```python
from build123d import *

# Parameters (mm, degrees)
PAD_DEPTH   = 40
SKETCH001_R = 7
HOLE_DEPTH  = 12.001


with BuildPart() as part:
    # Sketch → Pad (new body)
    with BuildSketch(Plane.XZ):
        Polygon((0, 0), (-18, 0), (-18, 7), (-13, 7), (-13, 2.5), (-10.5, 2.5), (-10.5, 9.5), (-20.5, 9.5), (-20.5, 12), (20.5, 12), (20.5, 9.5), (10.5, 9.5), (10.5, 2.5), (13, 2.5), (13, 7), (18, 7), (18, 0), align=None)
    extrude(amount=PAD_DEPTH)

    # Sketch001 (on Face9 of Pad) → Hole (cut, through all)
    with BuildSketch(Plane(origin=(0, 0, 12), x_dir=(-1, 0, 0), z_dir=(0, 0, 1))):
        with Locations((0, 20)):
            Circle(SKETCH001_R)
    extrude(amount=-HOLE_DEPTH, mode=Mode.SUBTRACT)


solid = part.part
```
Geometry check sheet. Reference: the model listing, model coordinates, mm. A direction names the side the tool comes from. Coordinates: 2 decimals unless noted, no trailing zeros. Order: outer loops, then holes, each group sorted by start corner. A loop starts at its lowest first (then second) coordinate and runs counter-clockwise, first axis right, second up.
Item 1: Depth check by flat-ended pin: pin 1 (1.5 mm diameter, centred on y = -7.5, z = 3, fed in from +X); pin 2 (2 mm diameter, centred on y = -24, z = 4, fed in from -X). Enter the tip coordinate at first touch or a pass-through.
Item 2: Section check C-C (x = -16). Enter the section's corners in (y, z), plus the area to 3 significant figures.
Item 3: Mould release check, pull along X, two halves, no side actions. Record for faces 1 (the flat face through (-10.5, -20, 6)), 2 (the flat face through (-8, -20, 0)), 3 (the flat face through (-20.5, -20, 11)): released by +X, released by -X, zero draft, split by the parting line, or undercut.
Item 4: Section check B-B (y = -20). Enter the section's corners in (x, z).
Item 5: Scan lines: line 1 along X through (y, z) = (-11.5, 3); line 2 along X through (y, z) = (-20, 6.75); line 3 along Z through (x, y) = (14, -6). Record each from-to range of solid material in increasing order.
Item 6: Tool access check on faces 4 (the flat face through (-16, -20, 7)), 5 (the flat face through (16, -20, 9.5)), 6 (the flat face through (18, -20, 4)), 7 (the flat face through (-13, -20, 5)). Record the directions out of +Z, -Z, +X, -X, +Y, -Y that give a thin tool (end or side, any length) a straight path to the whole face; none if there is none.
Item 7: Section check D-D (y = -7). Enter the section's corners in (x, z), plus the area to 4 significant figures.
Item 8: Section check A-A (z = 3.5). Enter the section's corners in (x, y).
Check sheet entries:
1. pin 1: stops at x = 18
1. pin 2: stops at x = -18
2. outline: (-40, 0) - (0, 0) - (0, 7) - (-40, 7) - close; (-40, 9.5) - (0, 9.5) - (0, 12) - (-40, 12) - close
2. area: 380 mm2
3. face 1: undercut
3. face 2: zero draft
3. face 3: released by -X
4. outline: (-20.5, 9.5) - (-10.5, 9.5) - (-10.5, 2.5) - (-13, 2.5) - (-13, 7) - (-18, 7) - (-18, 0) - (-7, 0) - (-7, 12) - (-20.5, 12) - close; (7, 0) - (18, 0) - (18, 7) - (13, 7) - (13, 2.5) - (10.5, 2.5) - (10.5, 9.5) - (20.5, 9.5) - (20.5, 12) - (7, 12) - close
5. line 1: x = -18 to -13, -10.5 to 10.5, 13 to 18
5. line 2: x = -18 to -13, -10.5 to -7, 7 to 10.5, 13 to 18
5. line 3: z = 0 to 7, 9.5 to 12
6. face 4: -X, +Y, -Y
6. face 5: +X, +Y, -Y
6. face 6: -Z, +X, +Y, -Y
6. face 7: +Y, -Y
7. outline: (-20.5, 9.5) - (-10.5, 9.5) - (-10.5, 2.5) - (-13, 2.5) - (-13, 7) - (-18, 7) - (-18, 0) - (18, 0) - (18, 7) - (13, 7) - (13, 2.5) - (10.5, 2.5) - (10.5, 9.5) - (20.5, 9.5) - (20.5, 12) - (-20.5, 12) - close
7. area: 384.5 mm2
8. outline: (-18, -40) - (-13, -40) - (-13, 0) - (-18, 0) - close; (-10.5, -40) - (10.5, -40) - (10.5, 0) - (-10.5, 0) - close; (13, -40) - (18, -40) - (18, 0) - (13, 0) - close; hole circle Ø14 at (0, -20)
